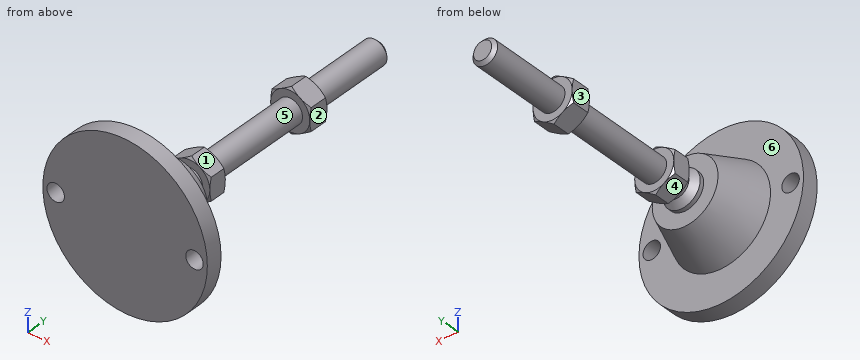
from build123d import *

# Parameters (mm, degrees)
EXTRUDE_1_DEPTH     = 9
EXTRUDE_2_DEPTH     = 10
SKETCH_5_R          = 4.25
CUT_EXTRUDE_1_DEPTH = 9


with BuildPart() as part:
    # Эскиз1 → Повернуть1 (revolve)
    with BuildSketch(Plane.XY, mode=Mode.PRIVATE) as revolve_1_sk:
        Polygon((0, 0), (-40, 0), (-40, 8), (-24, 8), (-16, 29), (-9, 29), (-9, 31), (-6, 34), (-6, 38), (-6, 47), (-6, 145.4), (-4.4, 147), (0, 147), align=None)
    revolve(revolve_1_sk.sketch.rotate(Axis((0, 0, 0), (0, 1, 0)), 180), axis=Axis((0, 0, 0), (0, 1, 0)))  # turned: the seam where the file's is

    # Эскиз2 → Бобышка-Вытянуть1 (add)
    with BuildSketch(Plane(origin=(0, 38, 0), x_dir=(1, 0, 0), z_dir=(0, 1, 0))):
        Polygon((0, 10.969655115), (-9.5, 5.484827557), (-9.5, -5.484827557), (0, -10.969655115), (9.5, -5.484827557), (9.5, 5.484827557), align=None)
    extrude(amount=EXTRUDE_1_DEPTH)

    # Эскиз3 → Бобышка-Вытянуть2 (add)
    with BuildSketch(Plane(origin=(0, 96.2, 0), x_dir=(1, 0, 0), z_dir=(0, 1, 0))):
        Polygon((9.5, 5.484827557), (0, 10.969655115), (-9.5, 5.484827557), (-9.5, -5.484827557), (0, -10.969655115), (9.5, -5.484827557), align=None)
    extrude(amount=EXTRUDE_2_DEPTH)

    # Эскиз4 → Вырез-Повернуть2 (revolve, cut)
    with BuildSketch(Plane.XY, mode=Mode.PRIVATE) as cut_revolve_2_sk:
        Polygon((-18.160254038, 106.2), (-9.5, 106.2), (-18.160254038, 101.2), align=None)
        Polygon((-18.160254038, 96.2), (-18.160254038, 101.2), (-9.5, 96.2), align=None)
        Polygon((-17.294228634, 47), (-17.294228634, 42.5), (-9.5, 47), align=None)
        Polygon((-17.294228634, 42.5), (-17.294228634, 38), (-9.5, 38), align=None)
    revolve(cut_revolve_2_sk.sketch.rotate(Axis((0, 147, 0), (0, -1, 0)), 180), axis=Axis((0, 147, 0), (0, -1, 0)), mode=Mode.SUBTRACT)  # turned: the seam where the file's is

    # Эскиз5 → Вырез-Вытянуть1 (cut, through all)
    with BuildSketch(Plane(origin=(0, 8, 0), x_dir=(1, 0, 0), z_dir=(0, 1, 0))):
        with Locations(Location((-33.75, 0, 0), (0, 0, 180))):  # turned: the seam where the file's is
            Circle(SKETCH_5_R)
        with Locations(Location((33.75, 0, 0), (0, 0, 180))):  # turned: the seam where the file's is
            Circle(SKETCH_5_R)
    extrude(amount=-CUT_EXTRUDE_1_DEPTH, mode=Mode.SUBTRACT)


solid = part.part
Build history of the part. All positions in model axes, mm. Face numbers are marked on the shaded views. A direction names the side the tool comes from. Round coordinates to 2 decimals unless told otherwise and drop trailing zeros. Write each loop counter-clockwise with the first axis right and the second up, starting at its lowest first coordinate (ties: lowest second). Pieces come first, ordered by that corner, then holes. Notation, with made-up numbers: (-24, 43) - (26, 43) arc R19 ccw to (26, 80) - close; hole circle Ø9 at (2, 43.5). An arc over 180 degrees is marked (long way). Use CSV: the item, a comma, the result in double quotes.
(1) Band-saw the part on A-A (x = 33.75). Write the cut outline in (y, z).
Response:
outline,"(0, -21.47) - (8, -21.47) - (8, -4.25) - (0, -4.25) - close; (0, 4.25) - (8, 4.25) - (8, 21.47) - (0, 21.47) - close"
(2) Band-saw the part on C-C (y = 17). Write the cut outline in (x, z), plus the area to 3 significant figures.
Response:
outline,"circle Ø41.14 at (0, 0)"
area,"1,330 mm²"
(3) Wall check: line 1 (Y direction, x = 1, z = -9); line 2 (Y direction, x = -2, z = -7); line 3 (Z direction, x = 33.75, y = 2.25). Give the ranges that are in metal, low to high.
Response:
line 1,"0 to 29, 38 to 47, 96.2 to 106.2"
line 2,"0 to 32.72, 38 to 47, 96.2 to 106.2"
line 3,"-21.47 to -4.25, 4.25 to 21.47"
(4) 3-axis set-ups, long thin cutter, end or side, ignore diameter. For the marked faces 1, 2 and 3: which of +Z, -Z, +X, -X, +Y, -Y reach the whole face in a straight line?
Response:
face 1,"+Z, +X, +Y"
face 2,"+Z, -Z, +X, +Y"
face 3,"+Z, -Z, -X, +Y"
(5) Band-saw the part on B-B (y = 51). Write the cut outline in (x, z).
Response:
outline,"circle Ø12 at (0, 0)"
(6) Mould opens along Y. For the marked faces 4, 5 and 6 say: pulls with the +Y half, pulls with the -Y half, needs draft (parallel to the pull), parting line crosses it, or undercut.
Response:
face 4,"needs draft"
face 5,"undercut"
face 6,"pulls with the +Y half"
(7) Pin check, flat tips, straight feed: P1, Ø3, axis at y = 101, z = -1, coming from the -X side; P2, Ø1, axis at x = 15.5, z = -21, coming from the +Y side; P3, Ø10, axis at y = 41, z = 2, coming from the +X side. Stop position of each tip, or through.
Response:
P1,"x = -9.5"
P2,"y = 8"
P3,"x = 9.5"
